Could you check a few things on this model? Use its own coordinates, in mm. Face numbers are marked on the shaded views. A direction names the side the tool comes from. Give positions to 0.01 mm unless a question says otherwise; leave off trailing zeros. Loops run counter-clockwise (first coordinate to the right, second up) from the corner with the lowest first, then second, coordinate; pieces in that order, holes last. Notation, with made-up numbers: (-1.5, 5.25) - (39.5, 5.25) arc R33 ccw to (39.5, 41.25) - close; hole circle Ø7 at (41, 72.25). An arc over 180 degrees is marked (long way). One line per item, written item: value. Start each with the question number.
Q1. I want a section at D-D (x = -21.5). Please give me the cut outline in (y, z).
Q2. If I drill on line 1 (Z direction, x = -11.5, y = -17.25); line 2 (Z direction, x = 10.5, y = -6); line 3 (Z direction, x = -18, y = -11.25), over which ranges is the centre line in solid material (lowest first)? Write a range as from..to.
Q3. If we mould it in two halves opening along Z, with no side actions, what happens to the marked faces 5, 6 and 7? For each: released by +Z, released by -Z, zero draft, split by the parting line, or undercut.
Q4. I want a section at B-B (x = 12). Please give me the cut outline in (y, z).
Q5. For the marked faces 1, 2, 3 and 4, which set-ups out of +Z, -Z, +X, -X, +Y, -Y let a thin tool reach every point of the face, with its end or its side?
Q6. I'm going to push flat-ended pins straight in: P1, Ø1.8, axis at x = 3.5, y = -11.5, coming from the +Z side; P2, Ø5.5, axis at x = -23.5, y = -17, coming from the -Z side; P3, Ø12, axis at x = -12.5, y = -8, coming from the +Z side. Where does each tip first touch, or does it pass through?
Q7. I want a section at C-C (z = -33). Please give me the cut outline in (x, y).
Q8. I want a section at A-A (z = 28). Please give me the cut outline in (x, y), then the cut area to 3 significant figures.
```python
from build123d import *

# Parameters (mm, degrees)
F1_DEPTH = 25.4


with BuildPart() as f1:
    # F0 (on Front) → F1 (new body)
    with BuildSketch(Plane.XZ):
        Polygon((-28.2575, -26.828751), (-13.652501, -26.828751), (-13.652501, -52.228753), (2.857499, -52.228753), (2.857499, -27.14625), (19.684996, -27.14625), (5.08, 5.87375), (19.684996, 5.87375), (2.857499, 36.036253), (9.207499, 36.036253), (-4.127499, 59.21375), (-19.685, 36.036253), (-10.16, 36.036253), (-28.2575, 5.87375), (-10.16, 5.87375), align=None)
        Polygon((-23.341425, 9.316429), (-13.652501, 23.902772), (-8.195201, 36.036253), (-8.195201, 38.463868), (-15.555656, 38.463868), (-8.195201, 50.051615), (-4.058297, 54.693776), (5.279458, 38.463868), (1.701662, 38.463868), (1.701662, 34.84314), (15.997937, 9.217735), (3.135762, 9.217735), (3.135762, 3.399133), (13.842684, -23.123091), (0, -23.123091), (0, -48.583038), (-11.602138, -48.583038), (-11.602138, -23.123091), (-23.341425, -23.123091), (-8.313072, 4.454316), (-8.313072, 9.316429), align=None, mode=Mode.SUBTRACT)
    extrude(amount=F1_DEPTH)


solid = f1.part
```
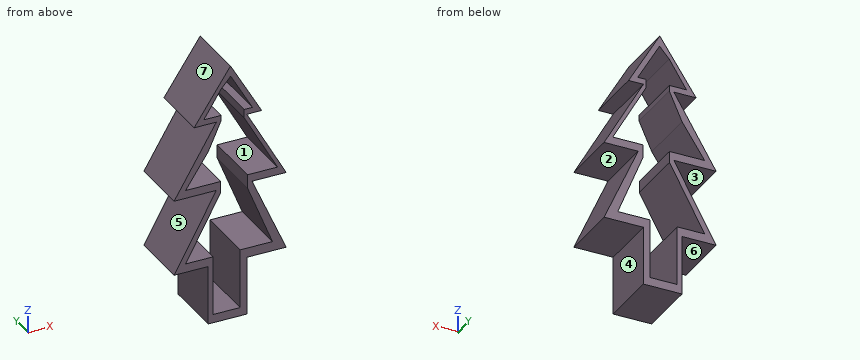
Worked answers:
1. outline: (-25.4, -26.83) - (0, -26.83) - (0, -23.12) - (-25.4, -23.12) - close; (-25.4, -19.74) - (0, -19.74) - (0, -14.62) - (-25.4, -14.62) - close; (-25.4, 5.87) - (0, 5.87) - (0, 9.32) - (-25.4, 9.32) - close; (-25.4, 12.09) - (0, 12.09) - (0, 17.14) - (-25.4, 17.14) - close
2. line 1: z = -52.23..-48.58, -1.39..3.45, 5.87..9.32, 28.69..33.8, 36.04..38.46, 44.85..48.23
2. line 2: z = -27.15..-23.12, -14.84..-6.38, 5.87..9.22, 19.07..22.34
2. line 3: z = -26.83..-23.12, -13.32..-8.29, 5.87..9.32, 17.36..22.97, 36.04..38.55
3. face 5: undercut
3. face 6: released by -Z
3. face 7: released by +Z
4. outline: (-25.4, -27.15) - (0, -27.15) - (0, -23.12) - (-25.4, -23.12) - close; (-25.4, -18.56) - (0, -18.56) - (0, -9.77) - (-25.4, -9.77) - close; (-25.4, 5.87) - (0, 5.87) - (0, 9.22) - (-25.4, 9.22) - close; (-25.4, 16.38) - (0, 16.38) - (0, 19.65) - (-25.4, 19.65) - close
5. face 1: +Y, -Y
5. face 2: +X, +Y, -Y
5. face 3: -X, +Y, -Y
5. face 4: -Z, +X, +Y, -Y
6. P1: stops at z = 47.52
6. P2: stops at z = -26.83
6. P3: stops at z = 55.68
7. outline: (-13.65, -25.4) - (-11.6, -25.4) - (-11.6, 0) - (-13.65, 0) - close; (0, -25.4) - (2.86, -25.4) - (2.86, 0) - (0, 0) - close
8. outline: (-14.98, -25.4) - (-11.81, -25.4) - (-11.81, 0) - (-14.98, 0) - close; (5.52, -25.4) - (7.34, -25.4) - (7.34, 0) - (5.52, 0) - close
8. area: 127 mm²
